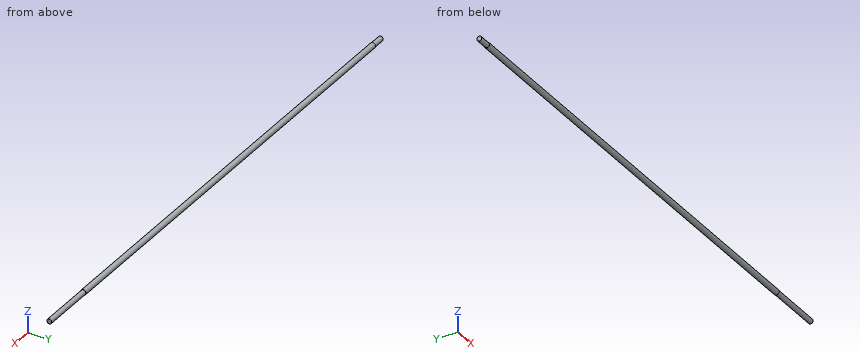
```python
from build123d import *

# Parameters (mm, degrees)
CYLINDER_R           = 5.556
CYLINDER_DEPTH       = 1066.8
CYLINDER_PITCH_ANGLE = 90
SKETCH_R             = 7
SKETCH_R_2           = 5
POCKET_DEPTH         = 25
SKETCH001_R          = 7
SKETCH001_R_2        = 5
POCKET001_DEPTH      = 110


with BuildPart() as part:
    # Cylinder → Cylinder (new body)
    with BuildSketch(Plane.XY):
        Circle(CYLINDER_R)
    extrude(amount=CYLINDER_DEPTH)


with BuildPart() as part_1:
    # Cylinder pitch: moved
    add(part.part.rotate(Axis((0, 0, 0), (0, 1, 0)), CYLINDER_PITCH_ANGLE))


with BuildPart() as part_2:
    # Cylinder placement: moved
    add(part_1.part.moved(Location((-491, -836, 778))))

    # Sketch → Pocket (cut)
    with BuildSketch(Plane(origin=(-491, -836, 778), x_dir=(0, 0, -1), z_dir=(-1, 0, 0))):
        Circle(SKETCH_R)
        Circle(SKETCH_R_2, mode=Mode.SUBTRACT)
    extrude(amount=-POCKET_DEPTH, mode=Mode.SUBTRACT)

    # Sketch001 → Pocket001 (cut)
    with BuildSketch(Plane(origin=(575.8, -836, 778), x_dir=(0, 0, -1), z_dir=(1, 0, 0))):
        Circle(SKETCH001_R)
        Circle(SKETCH001_R_2, mode=Mode.SUBTRACT)
    extrude(amount=-POCKET001_DEPTH, mode=Mode.SUBTRACT)


solid = part_2.part
```
Check sheet for the modelled part. Datum: model origin and axes. Units: mm. Round coordinates to 2 decimals unless told otherwise and drop trailing zeros. Order: outer loops, then holes, each group sorted by start corner. A loop starts at its lowest first (then second) coordinate and runs counter-clockwise, first axis right, second up. Notation, with made-up numbers: (89, -21.75) -> (131, -21.75) arc R29 cw to (131, 1.25) -> close; hole circle Ø7 at (77, 9). An arc over 180 degrees is marked (long way). One line per item, written item: value. Start each with the question number.
Q1. Cross-section at D-D (x = 488.5). Record the boundary of the cut face in (y, z).
Q2. Gauge pin test, flat ends, axial feed: pin 1 Ø2 at (x, y) = (46.5, -837.5) entering from +Z; pin 2 Ø3 at (x, y) = (257.5, -837.5) entering from +Z; pin 3 Ø1 at (x, y) = (151.5, -839) entering from -Z; pin 4 Ø2 at (x, y) = (-376.5, -840.5) entering from +Z (3 decimals). Record the tip position at first contact, or that the pin passes through.
Q3. Thickness scan on line 1 (Z direction, x = 102, y = -835); line 2 (Y direction, x = 162.5, z = 775.5); line 3 (Y direction, x = -93.5, z = 778.75). Record the ranges inside material, lowest first.
Q4. Cross-section at C-C (x = -81). Record the boundary of the cut face in (y, z), and give its area (3 significant figures).
Q5. Cross-section at B-B (y = -838.75). Record the boundary of the cut face in (x, z), and give its area (3 significant figures).
Q6. Cross-section at A-A (z = 780.25). Record the boundary of the cut face in (x, y).
Completed:
1. outline: circle Ø10 at (-836, 778)
2. pin 1: stops at z = 783.53
2. pin 2: stops at z = 783.56
2. pin 3: stops at z = 773.04
2. pin 4: stops at z = 782.315
3. line 1: z = 772.53 to 783.47
3. line 2: y = -840.96 to -831.04
3. line 3: y = -841.51 to -830.49
4. outline: circle Ø11.11 at (-836, 778)
4. area: 97.0 mm²
5. outline: (-491, 773.82) -> (-466, 773.82) -> (-466, 773.17) -> (465.8, 773.17) -> (465.8, 773.82) -> (575.8, 773.82) -> (575.8, 782.18) -> (465.8, 782.18) -> (465.8, 782.83) -> (-466, 782.83) -> (-466, 782.18) -> (-491, 782.18) -> close
5. area: 10,100 mm²
6. outline: (-491, -840.47) -> (-466, -840.47) -> (-466, -841.08) -> (465.8, -841.08) -> (465.8, -840.47) -> (575.8, -840.47) -> (575.8, -831.53) -> (465.8, -831.53) -> (465.8, -830.92) -> (-466, -830.92) -> (-466, -831.53) -> (-491, -831.53) -> close
